Work out the finished part from the listing and answer in its coordinate system (mm). Face numbers are marked on the shaded views. A direction names the side the tool comes from. Give positions to 0.01 mm unless a question says otherwise; leave off trailing zeros. Write each loop counter-clockwise with the first axis right and the second up, starting at its lowest first coordinate (ties: lowest second). Pieces come first, ordered by that corner, then holes. Notation, with made-up numbers: (-17, -14) -> (41, -14) arc R8 cw to (41, -1) -> close; hole circle Ø10 at (-37.75, -12). An arc over 180 degrees is marked (long way). Use a Markdown table: item, result. Add a question column.
Q1. Section C-C, the plane z = -13.5 is taken. Give the vertices of the cut face in (x, y).
Q2. Consider line 1 (Y direction, x = 9, z = -10); line 2 (X direction, y = 6.5, z = -6); line 3 (Z direction, x = 29, y = 5.1). Determine where each line is inside the solid, lowest interval first.
Q3. Section B-B, the plane x = 6 is taken. Give the vertices of the cut face in (y, z), plus the area to 3 significant figures.
Q4. For a pull along Y with two mould halves and no side action, classify the marked faces 1, 2 and 3 as pulls with the +Y half, pulls with the -Y half, needs draft (parallel to the pull), parting line crosses it, or undercut.
Q5. Each of these flat-tipped pins is pushed along its axis until it touches: pin 1 Ø1 at (y, z) = (-25, -19.5) entering from -X; pin 2 Ø1 at (y, z) = (-52, -8) entering from +X; pin 3 Ø8 at (x, y) = (12, -26.5) entering from +Z. Where does it stop, or does it pass through?
Q6. Section A-A, the plane z = -29 is taken. Give the vertices of the cut face in (x, y), plus the area to 3 significant figures.
Q7. Section D-D, the plane x = 11.5 is taken. Give the vertices of the cut face in (y, z), plus the area to 3 significant figures.
Q8. For the marked faces 4, 5, 6, 7 and 8, determine the directions among +Z, -Z, +X, -X, +Y, -Y from which every point of the face is accessible in a straight line to the end or side of a thin tool.
from build123d import *

# Parameters (mm, degrees)
SKETCH1_W           = 35
SKETCH1_H           = 35
BOSS_EXTRUDE1_DEPTH = 8
SKETCH2_W           = 5
SKETCH2_H           = 7
SKETCH2_W_2         = 7
SKETCH2_H_2         = 5
SKETCH2_R           = 1.5
CUT_EXTRUDE1_DEPTH  = 9
SKETCH2_5_R         = 4
SKETCH2_5_R_2       = 1.5
CUT_EXTRUDE2_DEPTH  = 4
SKETCH2_7_R         = 5
SKETCH2_7_R_2       = 2.5
BOSS_EXTRUDE2_DEPTH = 68
SKETCH3_W           = 18
SKETCH3_H           = 18
BOSS_EXTRUDE3_DEPTH = 4
FILLET1_R           = 5
SKETCH4_R           = 2.5
CUT_EXTRUDE3_DEPTH  = 10


with BuildPart() as part:
    # Sketch1 → Boss-Extrude1 (new body)
    with BuildSketch(Plane(origin=(0, 0, 0), x_dir=(1, 0, 0), z_dir=(0, 1, 0))):
        with Locations((17.5, 17.5)):
            Rectangle(SKETCH1_W, SKETCH1_H)
    extrude(amount=BOSS_EXTRUDE1_DEPTH)

    # Sketch2 → Cut-Extrude1 (cut, through all)
    with BuildSketch(Plane.XZ):
        with Locations((32.5, -21.5)):
            Rectangle(SKETCH2_W, SKETCH2_H)
        with Locations((13.5, -32.5)):
            Rectangle(SKETCH2_W_2, SKETCH2_H_2)
        with Locations((2.5, -13.5)):
            Rectangle(SKETCH2_W, SKETCH2_H)
        with Locations((21.5, -2.5)):
            Rectangle(SKETCH2_W_2, SKETCH2_H_2)
        with Locations((11, -11)):
            Circle(SKETCH2_R)
        with Locations((24, -11)):
            Circle(SKETCH2_R)
        with Locations((11, -24)):
            Circle(SKETCH2_R)
        with Locations((24, -24)):
            Circle(SKETCH2_R)
    extrude(amount=-CUT_EXTRUDE1_DEPTH, mode=Mode.SUBTRACT)

    # Sketch2_5 → Cut-Extrude2 (cut)
    with BuildSketch(Plane.XZ):
        with Locations((6, -29)):
            Circle(SKETCH2_5_R)
        with Locations((29, -6)):
            Circle(SKETCH2_5_R)
        with Locations((11, -11)):
            Circle(SKETCH2_5_R_2)
    extrude(amount=-CUT_EXTRUDE2_DEPTH, mode=Mode.SUBTRACT)

    # Sketch2_7 → Boss-Extrude2 (add)
    with BuildSketch(Plane.XZ):
        with Locations((17.5, -17.5)):
            Circle(SKETCH2_7_R)
        with Locations((29, -29)):
            Circle(SKETCH2_7_R_2)
        with Locations((6, -6)):
            Circle(SKETCH2_7_R_2)
    extrude(amount=BOSS_EXTRUDE2_DEPTH)

    # Sketch3 → Boss-Extrude3 (add)
    with BuildSketch(Plane(origin=(0, -68, 0), x_dir=(-1, 0, 0), z_dir=(0, -1, 0))):
        with Locations((-17.5, 17.5)):
            Rectangle(SKETCH3_W, SKETCH3_H)
    extrude(amount=BOSS_EXTRUDE3_DEPTH)

    # Fillet1
    fillet1_edges = [part.edges().sort_by_distance(p)[0] for p in [
        (0, 4, -35),
        (35, 4, -35),
        (35, 4, 0),
        (0, 4, 0),
    ]]
    fillet(fillet1_edges, radius=FILLET1_R)

    # Sketch4 → Cut-Extrude3 (cut)
    with BuildSketch(Plane(origin=(0, 4, 0), x_dir=(-1, 0, 0), z_dir=(0, -1, 0))):
        with Locations((-29, 6)):
            Circle(SKETCH4_R)
        with Locations((-6, 29)):
            Circle(SKETCH4_R)
    extrude(amount=-CUT_EXTRUDE3_DEPTH, mode=Mode.SUBTRACT)


solid = part.part
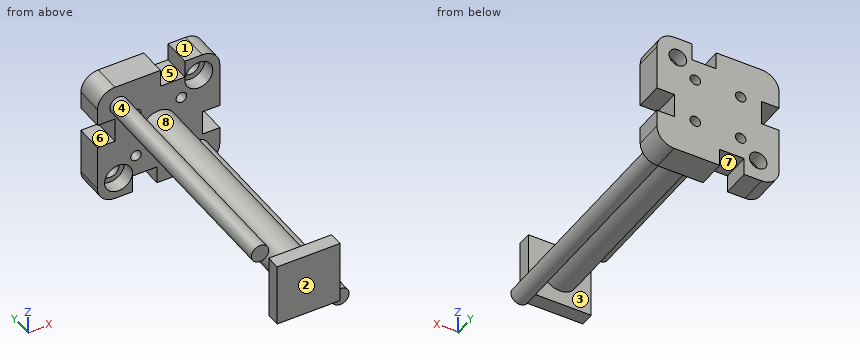
Result set:
| question | item | result |
|---|---|---|
| 1 | outline | (5, 0) -> (14.5, 0) -> (14.5, -68) -> (8.5, -68) -> (8.5, -72) -> (26.5, -72) -> (26.5, -68) -> (20.5, -68) -> (20.5, 0) -> (35, 0) -> (35, 8) -> (5, 8) -> close |
| 2 | line 1 | y = -72 to -68, 0 to 8 |
| 2 | line 2 | x = 0 to 26.5, 31.5 to 35 |
| 2 | line 3 | z = -35 to -8.5, -3.5 to 0 |
| 3 | outline | (-68, -8.5) -> (0, -8.5) -> (0, -25) -> (4, -25) -> (4, -26.5) -> (8, -26.5) -> (8, 0) -> (0, 0) -> (0, -3.5) -> (-68, -3.5) -> close; (0, -35) -> (8, -35) -> (8, -31.5) -> (4, -31.5) -> (4, -33) -> (0, -33) -> close |
| 3 | area | 568 mm2 |
| 4 | face 1 | needs draft |
| 4 | face 2 | pulls with the -Y half |
| 4 | face 3 | undercut |
| 5 | pin 1 | stops at x = 12.73 |
| 5 | pin 2 | stops at x = 8 |
| 5 | pin 3 | stops at z = -4.5 |
| 6 | outline | (0, 0) -> (2, 0) -> (2, 4) -> (3.5, 4) -> (3.5, 8) -> (0, 8) -> close; (8.5, 4) -> (10, 4) -> (10, 0) -> (26.5, 0) -> (26.5, -68) -> (31.5, -68) -> (31.5, 0) -> (35, 0) -> (35, 8) -> (8.5, 8) -> close |
| 6 | area | 568 mm2 |
| 7 | outline | (-72, -26.5) -> (-68, -26.5) -> (-68, -8.5) -> (-72, -8.5) -> close; (0, -30) -> (8, -30) -> (8, -25.41) -> (0, -25.41) -> close; (0, -22.59) -> (8, -22.59) -> (8, -12.41) -> (0, -12.41) -> close; (0, -9.59) -> (8, -9.59) -> (8, 0) -> (0, 0) -> close |
| 7 | area | 267 mm2 |
| 8 | face 4 | -Y |
| 8 | face 5 | +Z, +Y, -Y |
| 8 | face 6 | -X, +Y, -Y |
| 8 | face 7 | -Z, +Y, -Y |
| 8 | face 8 | none |
